```python
from build123d import *

# Parameters (mm, degrees)
PAD014_DEPTH    = 28.8
POCKET011_DEPTH = 24
POCKET012_DEPTH = 24
SKETCH112_W     = 2
SKETCH112_H     = 16
POCKET028_DEPTH = 30
PAD141_DEPTH    = 22
PAD142_DEPTH    = 24
POCKET056_DEPTH = 24
POCKET057_DEPTH = 23
SKETCH194_W     = 16
SKETCH194_H     = 2
POCKET076_DEPTH = 30


with BuildPart() as part:
    # Sketch025 (on Face52 of Binder010) → Pad014 (new body)
    with BuildSketch(Plane.XY.offset(-28.8)):
        Polygon((0, 0), (0, 8), (-16, 8), (-16, -16), (8, -16), (8, 0), align=None)
    extrude(amount=PAD014_DEPTH)

    # Sketch026 (on Face5 of Pad014) → Pocket011 (cut)
    with BuildSketch(Plane.YZ.offset(8)):
        Polygon((-16, -9.6), (0, 0), (-16, 0), align=None)
    extrude(amount=-POCKET011_DEPTH, mode=Mode.SUBTRACT)

    # Sketch027 (on Face3 of Pocket011) → Pocket012 (cut)
    with BuildSketch(Plane(origin=(0, 8, 0), x_dir=(-1, 0, 0), z_dir=(0, 1, 0))):
        Polygon((16, -9.6), (0, 0), (16, 0), align=None)
    extrude(amount=-POCKET012_DEPTH, mode=Mode.SUBTRACT)

    # Sketch112 (on Face4 of Pocket012) → Pocket028 (cut)
    with BuildSketch(Plane(origin=(0, 0, -28.8), x_dir=(1, 0, 0), z_dir=(0, 0, -1))):
        with Locations((7, 8)):
            Rectangle(SKETCH112_W, SKETCH112_H)
    extrude(amount=-POCKET028_DEPTH, mode=Mode.SUBTRACT)

    # Sketch137 (on Face7 of Pocket028) → Pad141 (join)
    with BuildSketch(Plane.YZ.offset(6)):
        Polygon((0, 0), (-3.2, 0), (-16, -7.68), (-16, -10.88), (-3.2, -3.2), (0, -3.2), align=None)
    extrude(amount=-PAD141_DEPTH)

    # Sketch167 → Pad142 (join)
    with BuildSketch(Plane(origin=(0, 8, 0), x_dir=(-1, 0, 0), z_dir=(0, 1, 0))):
        Polygon((0, 0), (0, -3.2), (3.2, -3.2), (16, -10.88), (16, -7.68), (3.2, 0), align=None)
    extrude(amount=-PAD142_DEPTH)

    # Sketch170 (on Face9 of Pad142) → Pocket056 (cut)
    with BuildSketch(Plane(origin=(0, 8, 0), x_dir=(-1, 0, 0), z_dir=(0, 1, 0))):
        Polygon((3.2, 0), (16, -7.68), (16, 0), align=None)
    extrude(amount=-POCKET056_DEPTH, mode=Mode.SUBTRACT)

    # Sketch171 (on Face3 of Pocket056) → Pocket057 (cut)
    with BuildSketch(Plane.YZ.offset(6)):
        Polygon((-3.2, 0), (-16, -7.68), (-16, 0), align=None)
    extrude(amount=-POCKET057_DEPTH, mode=Mode.SUBTRACT)

    # Sketch194 (on Face1 of Pocket057) → Pocket076 (cut)
    with BuildSketch(Plane(origin=(0, 0, -28.8), x_dir=(1, 0, 0), z_dir=(0, 0, -1))):
        with Locations((-8, -7)):
            Rectangle(SKETCH194_W, SKETCH194_H)
    extrude(amount=-POCKET076_DEPTH, mode=Mode.SUBTRACT)


solid = part.part
```
Work out the finished part from the listing and answer in its coordinate system (mm). A direction names the side the tool comes from. Round coordinates to 2 decimals unless told otherwise and drop trailing zeros. Loops run counter-clockwise (first coordinate to the right, second up) from the corner with the lowest first, then second, coordinate; pieces in that order, holes last. Notation, with made-up numbers: M 84.5,-30.5 L 136.5,-30.5 A22 cw 136.5,-9.5 Z; hole C 63,65 d1. An arc over 180 degrees is marked long. Use CSV: the item, a comma, the result in double quotes.
Q1. Consider L1, parallel to X at y = 4.75, z = -24.75; L2, parallel to Z at x = -4.25, y = -5.75. Determine where each line is inside the solid, lowest interval first.
Determined:
L1,"-16 to 0"
L2,"-28.8 to -1.53"
Q2. Section B-B, the plane y = -7.5 is taken. Determine the outline of the cut face in (x, z), then the cut area to 3 significant figures.
Determined:
outline,"M -16,-28.8 L 6,-28.8 L 6,-2.58 L -7.5,-2.58 L -16,-7.68 Z"
area,"555 mm2"
Q3. Each of these flat-tipped pins is pushed along its axis until it touches: pin 1 (6 mm diameter, centred on x = -10, y = 3, fed in from +Z); pin 2 (3 mm diameter, centred on y = 4, z = -10.5, fed in from +X); pin 3 (3 mm diameter, centred on x = 3, z = -16, fed in from +Y). Where does it stop, or does it pass through?
Determined:
pin 1,"z = -2.28"
pin 2,"x = 0"
pin 3,"y = 0"
Q4. Section C-C, the plane z = -8.25 is taken. Determine the outline of the cut face in (x, y).
Determined:
outline,"M -16,-16 L 6,-16 L 6,0 L 0,0 L 0,6 L -16,6 Z"
Q5. A tool of negligible diameter and unlimited length cuts with its end or side. For faces 1 (the flat face through (3, 0, -15)), 2 (the flat face through (-16, -5, -18)), from which of +Z, -Z, +X, -X, +Y, -Y can it reach the whole face along a straight path? Write none if from no direction.
Determined:
face 1,"+Z, -Z, +X, +Y"
face 2,"+Z, -Z, -X, +Y, -Y"
Q6. Section D-D, the plane z = -5 is taken. Determine the outline of the cut face in (x, y), then the cut area to 3 significant figures.
Determined:
outline,"M -11.53,-11.53 L 6,-11.53 L 6,0 L 0,0 L 0,6 L -11.53,6 Z"
area,"271 mm2"
Q7. Section A-A, the plane x = -2.25 is taken. Determine the outline of the cut face in (y, z), then the cut area to 3 significant figures.
Determined:
outline,"M -16,-28.8 L 6,-28.8 L 6,0 L -3.2,0 L -16,-7.68 Z"
area,"584 mm2"
